The model under review builds one solid part; all positions refer to its coordinate system, in mm. Face numbers are marked on the shaded views. Coordinates: 2 decimals unless noted, no trailing zeros. Write each loop counter-clockwise with the first axis right and the second up, starting at its lowest first coordinate (ties: lowest second). Pieces come first, ordered by that corner, then holes. Notation, with made-up numbers: (86.25, 6.5) - (116.25, 6.5) arc R28 cw to (116.25, 44.5) - close; hole circle Ø2 at (-31, -12.5). An arc over 180 degrees is marked (long way). Put each result on its own line as item: value. Start each with the question number.
Item 1: To check wall thickness, follow L1, parallel to Z at x = 0, y = 0.2; L2, parallel to Y at x = 1.5, z = -4. State the ranges of each line that lie inside material, in increasing order. Write a range as [from, to].
Item 2: Consider section D-D on z = 3.25. Give the boundary of the cut face in (x, y).
Item 3: Consider section B-B on x = 0. Give the boundary of the cut face in (y, z).
Item 4: Consider section A-A on z = 0. Give the boundary of the cut face in (x, y), then the cut area to 3 significant figures.
Item 5: Consider section C-C on y = 0.4. Give the boundary of the cut face in (x, z).
Item 6: For pin 1 (2 mm diameter, centred on x = -1, z = 2, fed in from +Y), flat-tipped, find the tip position at first contact; note if it passes through.
Item 7: Mouldability with a two-part tool opening along Y and no side actions: class the marked faces 1, 2, 3 and 4 as pulls with the +Y half, pulls with the -Y half, needs draft (parallel to the pull), parting line crosses it, or undercut.
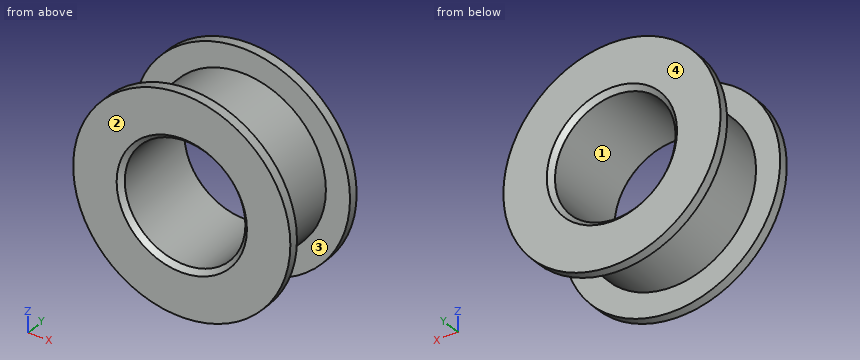
Autodesk Inventor part; units mm, degrees
ref_plane "YZ Plane" through (0, 0, 0) normal (1, 0, 0) x (0, 1, 0)
ref_plane "XZ Plane" through (0, 0, 0) normal (0, 1, 0) x (-1, 0, 0)
ref_plane "XY Plane" through (0, 0, 0) normal (0, 0, 1) x (1, 0, 0)
sketch "Skizze1" plane through (0, 0, 0) normal (0, 0, 1) x (1, 0, 0)
  line L0 (0, -2) -> (0, 2)
  line L1 (2.5, 2) -> (2.5, -2)
  line L2 (4.5, -2) -> (4.5, -1.6)
  line L3 (4.5, -1.6) -> (3.5, -1.6)
  line L4 (3.5, -1.6) -> (3.5, 1.6)
  line L5 (3.5, 1.6) -> (4.5, 1.6)
  line L6 (4.5, 1.6) -> (4.5, 2)
  line L7 (-0.9, 0) -> (5.4, 0)
  line L8 (4.5, -2) -> (2.5, -2)
  line L9 (4.5, 2) -> (2.5, 2)
  point P0 (0, 0)
  point P1 (0, 0)
  dimension "d0" = 5
  dimension "d3" = 7
  dimension "d4" = 1
  dimension "d6" = 4
  dimension "d8" = 3.2
revolve "Umdrehung1" add sketch "Skizze1" angle 360 about axis through (0, -2, 0) along (0, 1, 0)
chamfer "Fase2" distance 0.2 angle 45 2 edges at (-2.5, 2, 0) (-2.5, -2, 0)
properties part number "Rolle" material "Aluminium 6061"
Report:
1. L1: [-3.5, -2.5], [2.5, 3.5]
1. L2: [-2, -1.6], [1.6, 2]
2. outline: (-3.11, -2) - (3.11, -2) - (3.11, -1.6) - (1.3, -1.6) - (1.3, 1.6) - (3.11, 1.6) - (3.11, 2) - (-3.11, 2) - (-3.11, 1.6) - (-1.3, 1.6) - (-1.3, -1.6) - (-3.11, -1.6) - close
3. outline: (-2, -4.5) - (-1.6, -4.5) - (-1.6, -3.5) - (1.6, -3.5) - (1.6, -4.5) - (2, -4.5) - (2, -2.7) - (1.8, -2.5) - (-1.8, -2.5) - (-2, -2.7) - close; (-2, 2.7) - (-1.8, 2.5) - (1.8, 2.5) - (2, 2.7) - (2, 4.5) - (1.6, 4.5) - (1.6, 3.5) - (-1.6, 3.5) - (-1.6, 4.5) - (-2, 4.5) - close
4. outline: (-4.5, -2) - (-2.7, -2) - (-2.5, -1.8) - (-2.5, 1.8) - (-2.7, 2) - (-4.5, 2) - (-4.5, 1.6) - (-3.5, 1.6) - (-3.5, -1.6) - (-4.5, -1.6) - close; (2.5, -1.8) - (2.7, -2) - (4.5, -2) - (4.5, -1.6) - (3.5, -1.6) - (3.5, 1.6) - (4.5, 1.6) - (4.5, 2) - (2.7, 2) - (2.5, 1.8) - close
4. area: 9.52 mm²
5. outline: circle Ø7 at (0, 0); hole circle Ø5 at (0, 0)
6. pin 1: y = 2
7. face 1: needs draft
7. face 2: pulls with the -Y half
7. face 3: undercut
7. face 4: pulls with the +Y half
